Autodesk Inventor part; units mm, degrees
ref_plane "YZ Plane" through (0, 0, 0) normal (1, 0, 0) x (0, 1, 0)
ref_plane "XZ Plane" through (0, 0, 0) normal (0, 1, 0) x (-1, 0, 0)
ref_plane "XY Plane" through (0, 0, 0) normal (0, 0, 1) x (1, 0, 0)
sketch "草图1" plane through (0, 0, 0) normal (0, 0, 1) x (1, 0, 0)
  circle A0 centre (0, 0) radius 15
  dimension "d0" = 30
extrude "拉伸1" add sketch "草图1" along normal blind 25
sketch "草图2" plane through (0, 0, 25) normal (0, 0, 1) x (1, 0, 0)
  circle A0 centre (0, 0) radius 10
  dimension "d3" = 20
extrude "拉伸2" cut sketch "草图2" against normal blind 20
thread "螺纹1"
sketch "草图3" plane through (0, 0, 0) normal (0, 0, -1) x (-1, 0, 0)
  line L0 (10, 5.7735) -> (10, -5.7735)
  line L1 (10, -5.7735) -> (0, -11.547)
  line L2 (0, -11.547) -> (-10, -5.7735)
  line L3 (-10, -5.7735) -> (-10, 5.7735)
  line L4 (-10, 5.7735) -> (0, 11.547)
  line L5 (0, 11.547) -> (10, 5.7735)
  line L6 (0, 0) -> (-10, 0)
  dimension "d8" = 20
extrude "拉伸3" add sketch "草图3" along normal blind 8
fillet "圆角1" radius 1 13 edges at (-15, 0, 0) (5, 8.6603, -8) (-5, 8.6603, -8) (-10, 0, -8) (-5, -8.6603, -8) (5, -8.6603, -8) (10, 0, -8) (10, 5.7735, -4) (0, 11.547, -4) (-10, 5.7735, -4) (-10, -5.7735, -4) (0, -11.547, -4) (10, -5.7735, -4)
properties part number "水箱出水口盖"
Here's how the part is built. I have some questions about the finished solid (model axes, mm). A direction names the side the tool comes from. Round coordinates to 2 decimals unless told otherwise and drop trailing zeros. Order: outer loops, then holes, each group sorted by start corner. A loop starts at its lowest first (then second) coordinate and runs counter-clockwise, first axis right, second up. Notation, with made-up numbers: (17.25, 39.5) -> (71.25, 39.5) arc R20 ccw to (71.25, 64.5) -> close; hole circle Ø6 at (1, 27). An arc over 180 degrees is marked (long way). Return JSON: item names as keys, results as strings.
Q1. For pin 1 Ø7.5 at (y, z) = (-2.5, -4.5) entering from -X; pin 2 Ø10 at (x, y) = (4.5, 5) entering from +Z; pin 3 Ø12 at (x, y) = (0, 0) entering from +Z; pin 4 Ø8 at (y, z) = (-5.5, 12) entering from -X, each with a flat end and sliding along its axis, tell me the tip position at first contact or that it passes through.
Filled sheet:
{"pin 1": "stops at x = -10", "pin 2": "stops at z = 25", "pin 3": "stops at z = 5", "pin 4": "stops at x = -14.92"}
Q2. If we section it at A-A on y = 0: List the corners of the cut face in (x, z) for me.
Filled sheet:
{"outline": "(-15, 1) arc R1 ccw to (-14, 0) -> (-10, 0) -> (-10, -7) arc R1 ccw to (-9, -8) -> (9, -8) arc R1 ccw to (10, -7) -> (10, 0) -> (14, 0) arc R1 ccw to (15, 1) -> (15, 25) -> (10, 25) -> (10, 5) -> (-10, 5) -> (-10, 25) -> (-15, 25) -> close"}
Q3. If we section it at B-B on z = -4: List the corners of the cut face in (x, y) for me.
Filled sheet:
{"outline": "(-10, -5.2) arc R1 ccw to (-9.5, -6.06) -> (-0.5, -11.26) arc R1 ccw to (0.5, -11.26) -> (9.5, -6.06) arc R1 ccw to (10, -5.2) -> (10, 5.2) arc R1 ccw to (9.5, 6.06) -> (0.5, 11.26) arc R1 ccw to (-0.5, 11.26) -> (-9.5, 6.06) arc R1 ccw to (-10, 5.2) -> close"}
Q4. I need wall thicknesses on line 1 along Y through (x, z) = (0, 10); line 2 along Y through (x, z) = (12, 19); line 3 along X through (y, z) = (-0.5, 1). Which ranges of each line are inside material? Lowest first, please. Write a range as from..to.
Filled sheet:
{"line 1": "y = -15..-10, 10..15", "line 2": "y = -9..9", "line 3": "x = -14.99..14.99"}
Q5. If we section it at C-C on z = 9.5: List the corners of the cut face in (x, y) for me.
Filled sheet:
{"outline": "circle Ø30 at (0, 0); hole circle Ø20 at (0, 0)"}
Q6. If we mould it in two halves opening along Y, with no side actions, what happens to faces 1 (the cylindrical face through (-2.17, -9.76, 15.14)), 2 (the cylindrical face through (9.87, -5.69, -3.55)), 3 (the flat face through (0, 0, -8)), 4 (the cylindrical face through (-9.87, 5.69, -3.55))? For each: released by +Y, released by -Y, zero draft, split by the parting line, or undercut.
Filled sheet:
{"face 1": "undercut", "face 2": "released by -Y", "face 3": "zero draft", "face 4": "released by +Y"}
Q7. Which directions (+Z, -Z, +X, -X, +Y, -Y) give clear straight access to the entire face, cutting with the end or side of a thin tool? Please do faces 5 (the flat face through (-5.063, -8.624, -3.451)), 6 (the flat face through (10, 0, -3)), 7 (the flat face through (-4.937, 8.697, -3.451)).
Filled sheet:
{"face 5": "-Z, -X, -Y", "face 6": "-Z, +X, +Y, -Y", "face 7": "-Z, -X, +Y"}
